Job drawing, mm, ordinate dimensions from the low corner. One solid piece. A direction names the side the tool comes from. Coordinates: 2 decimals unless noted, no trailing zeros. Loops run counter-clockwise (first coordinate to the right, second up) from the corner with the lowest first, then second, coordinate; pieces in that order, holes last. Notation, with made-up numbers: M 32,-32 L 75,-32 A11 cw 75,-24 Z; hole C -6.5,38 d5. An arc over 180 degrees is marked long. Answer as a JSON object with one key per item and string values. Group by question number.
1. Drill centre lines: L1, parallel to Z at x = 17, y = 1.8; L2, parallel to Y at x = 30, z = 33; L3, parallel to X at y = 4.5, z = 7. Where is each one in solid material? Low to high.
2. 3-axis set-ups, long thin cutter, end or side, ignore diameter. For the marked faces 1, 2 and 3: which of +Z, -Z, +X, -X, +Y, -Y reach the whole face in a straight line?
3. Saw through at D-D on y = 16. Write the cut outline in (x, z).
4. Saw through at C-C on z = 23. Write the cut outline in (x, y).
5. Saw through at B-B on z = 9. Write the cut outline in (x, y), then the cut area to 3 significant figures.
6. Saw through at A-A on x = 17. Write the cut outline in (y, z), then the cut area to 3 significant figures.
7. Drop flat-ended pins along their axis: pin 1 Ø12 at (x, z) = (15, 18.5) entering from +Y; pin 2 Ø6 at (x, z) = (38.5, 30.5) entering from -Y; pin 3 Ø6.5 at (y, z) = (15, 12.5) entering from +X. Give the stop position or say it passes through.
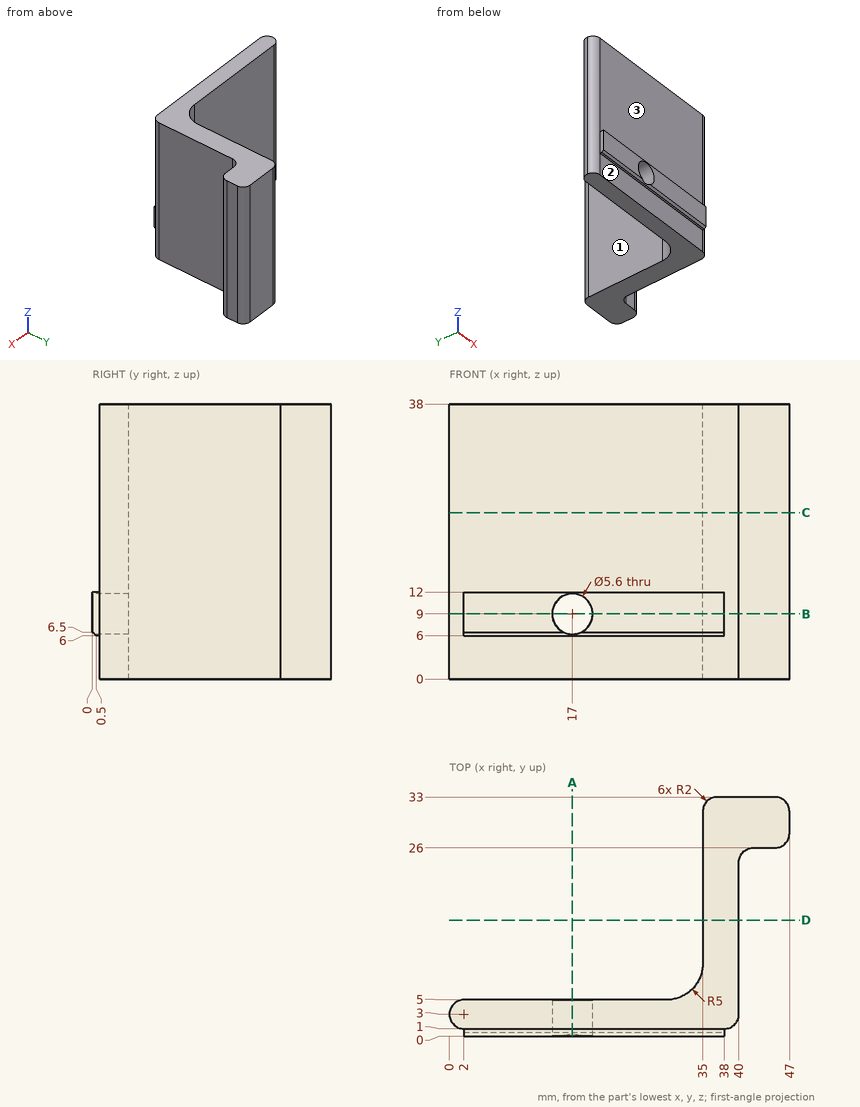
Outcome:
{
 "1": {"L1": "z = 0 to 6.2, 11.8 to 38", "L2": "y = 1 to 5", "L3": "x = 0.68 to 15.04, 18.96 to 40"},
 "2": {"face 1": "+Z, -Z, -X, +Y", "face 2": "-Z, +X, -X, -Y", "face 3": "+Z, +X, -X, -Y"},
 "3": {"outline": "M 35,0 L 40,0 L 40,38 L 35,38 Z"},
 "4": {"outline": "M 2,1 L 38,1 A2 ccw 40,3 L 40,24 A2 cw 42,26 L 45,26 A2 ccw 47,28 L 47,31 A2 ccw 45,33 L 37,33 A2 ccw 35,31 L 35,10 A5 cw 30,5 L 2,5 A2 ccw Z"},
 "5": {"outline": "M 2,0 L 14.2,0 L 14.2,5 L 2,5 A2 ccw 2,1 Z; M 19.8,0 L 38,0 L 38,1 A2 ccw 40,3 L 40,24 A2 cw 42,26 L 45,26 A2 ccw 47,28 L 47,31 A2 ccw 45,33 L 37,33 A2 ccw 35,31 L 35,10 A5 cw 30,5 L 19.8,5 Z", "area": "358 mm²"},
 "6": {"outline": "M 0,11.8 L 5,11.8 L 5,38 L 1,38 L 1,12 L 0,12 Z; M 0.3,6.2 L 0.5,6 L 1,6 L 1,0 L 5,0 L 5,6.2 Z", "area": "130 mm²"},
 "7": {"pin 1": "stops at y = 5", "pin 2": "stops at y = 1", "pin 3": "stops at x = 40"}
}
